```python
from build123d import *

# Parameters (mm, degrees)
SKETCH1_W           = 8.784371833
SKETCH1_H           = 3.000075643
BOSS_EXTRUDE1_DEPTH = 3.175


with BuildPart() as part:
    # Sketch1 → Boss-Extrude1 (new body)
    with BuildSketch(Plane(origin=(0, 0, 0), x_dir=(1, 0, 0), z_dir=(0, 1, 0))):
        with BuildLine():
            add(Edge.make_bspline(
                [(-28.61031783, -15.731991288), (-28.599265415, -13.470035002), (-28.589694066, -11.351623557)],
                knots=[4, 4, 4, 4.067001907, 4.067001907, 4.067001907], degree=2))
            Line((-28.61031783, -15.731991288), (-26.367380226, -15.731991288))
            Line((-26.367380226, -15.731991288), (-26.367380226, -12.731847281))
            Line((-26.367380226, -12.731847281), (-24.870018528, -12.731847281))
            Line((-24.870018528, -12.731847281), (-24.870018528, -15.731991288))
            Line((-24.870018528, -15.731991288), (-22.620949028, -15.731991288))
            Line((-22.620949028, -15.731991288), (-22.620949028, -12.731847281))
            Line((-22.620949028, -12.731847281), (-20.62449601, -12.731847281))
            Line((-20.62449601, -12.731847281), (-20.62449601, -8.731700034))
            Line((-20.62449601, -8.731700034), (-21.872234059, -8.731700034))
            Line((-21.872234059, -8.731700034), (-21.872234059, -8.631722416))
            Line((-21.872234059, -8.631722416), (-21.872234059, -6.131583692))
            Line((-21.872234059, -6.131583692), (-20.62449601, -6.131583692))
            Line((-20.62449601, -6.131583692), (-20.62449601, -2.631434402))
            Line((-20.62449601, -2.631434402), (-17.629967586, -2.631434402))
            Line((-17.629967586, -2.631434402), (-17.629967586, -6.131583692))
            Line((-17.629967586, -6.131583692), (-16.382151548, -6.131583692))
            Line((-16.382151548, -6.131583692), (-16.382151548, -8.631722416))
            Line((-16.382151548, -8.631722416), (-16.382151548, -8.731700034))
            Line((-16.382151548, -8.731700034), (-17.629967586, -8.731700034))
            Line((-17.629967586, -8.731700034), (-17.629967586, -12.731847281))
            Line((-17.629967586, -12.731847281), (-13.936374012, -12.731847281))
            Line((-13.936374012, -12.731847281), (-13.936374012, -15.731991288))
            Line((-13.936374012, -15.731991288), (-9.644077522, -15.731991288))
            Line((-9.644077522, -15.731991288), (-9.644077522, 32.969811886))
            Line((-9.644077522, 32.969811886), (-12.638791169, 32.969811886))
            Line((-12.638791169, 32.969811886), (-12.638791169, 35.969951009))
            Line((-12.638791169, 35.969951009), (-15.633504817, 35.969951009))
            Line((-15.633504817, 35.969951009), (-15.633504817, 32.969811886))
            Line((-15.633504817, 32.969811886), (-17.629967584, 32.969811886))
            Line((-17.629967584, 32.969811886), (-17.629967584, 29.869690261))
            Line((-17.629967584, 29.869690261), (-16.382151546, 29.869690261))
            Line((-16.382151546, 29.869690261), (-16.382151546, 27.369615017))
            Line((-16.382151546, 27.369615017), (-17.629967584, 27.369615017))
            Line((-17.629967584, 27.369615017), (-17.629967584, 23.569352199))
            Line((-17.629967584, 23.569352199), (-20.624496008, 23.569352199))
            Line((-20.624496008, 23.569352199), (-20.624496008, 27.369615017))
            Line((-20.624496008, 27.369615017), (-21.872234057, 27.369615017))
            Line((-21.872234057, 27.369615017), (-21.872234057, 29.869690261))
            Line((-21.872234057, 29.869690261), (-20.624496008, 29.869690261))
            Line((-20.624496008, 29.869690261), (-20.624496008, 32.969811886))
            Line((-20.624496008, 32.969811886), (-22.620949026, 32.969811886))
            Line((-22.620949026, 32.969811886), (-22.620949026, 35.969951009))
            Line((-22.620949026, 35.969951009), (-24.870018526, 35.969951009))
            Line((-24.870018526, 35.969951009), (-24.870018526, 32.969811886))
            Line((-24.870018526, 32.969811886), (-26.367380224, 32.969811886))
            Line((-26.367380224, 32.969811886), (-26.367380224, 35.969951009))
            Line((-26.367380224, 35.969951009), (-28.610317827, 35.969951009))
            Line((-28.610317827, 35.969951009), (-28.610317827, 31.489897526))
            add(Edge.make_bspline(
                [(-24.079715861, 26.005231108), (-24.142399609, 31.393191619), (-26.553744953, 31.462825341), (-28.610317827, 31.489897526)],
                knots=[6, 6, 6, 6, 7, 7, 7, 7], degree=3))
            add(Edge.make_bspline(
                [(-28.610317828, 19.811970764), (-26.367380222, 19.876359983), (-24.017041861, 20.617148519), (-24.079715861, 26.005231108)],
                knots=[5, 5, 5, 5, 6, 6, 6, 6], degree=3))
            add(Edge.make_bspline(
                [(-28.542036738, 1.284383122), (-28.493620066, 18.549619675), (-28.610317828, 19.811970764)],
                knots=[4.292555269, 4.292555269, 4.292555269, 5, 5, 5], degree=2))
            add(Edge.make_bspline(
                [(-28.542036738, 1.284383122), (-26.304598455, 1.216834034), (-24.092636702, 0.462074592), (-24.122268671, -5.143929938)],
                knots=[1.002428408, 1.002428408, 1.002428408, 1.002428408, 2, 2, 2, 2], degree=3))
            add(Edge.make_bspline(
                [(-24.122268671, -5.143929938), (-24.151883253, -10.744553605), (-26.537723417, -11.321030016), (-28.589694066, -11.351623557)],
                knots=[2, 2, 2, 2, 2.996659117, 2.996659117, 2.996659117, 2.996659117], degree=3))
        make_face()
        with Locations((-19.726124806, 7.868969519)):
            Rectangle(SKETCH1_W, SKETCH1_H, mode=Mode.SUBTRACT)
    extrude(amount=BOSS_EXTRUDE1_DEPTH)


solid = part.part
```
CAD build for the part. Positions are in the model's coordinates, mm. A direction names the side the tool comes from. Round coordinates to 2 decimals unless told otherwise and drop trailing zeros. Order: outer loops, then holes, each group sorted by start corner. A loop starts at its lowest first (then second) coordinate and runs counter-clockwise, first axis right, second up. Notation, with made-up numbers: (0.5, 86.25) - (8.5, 86.25) arc R21 cw to (8.5, 108.25) - close; hole circle Ø4 at (55, 54). An arc over 180 degrees is marked (long way). Answer as CSV lines item,"result". Start each with the question number.
1. Saw through at D-D, the plane x = -27. Count the separate pieces of the cut face and the enclosed holes in it, and give its area (3 significant figures).
2. Saw through at C-C, the plane x = -11.25. Write the cut outline in (y, z) (3 decimals).
3. Saw through at B-B, the plane x = -23.25. Write the cut outline in (y, z) (3 decimals), and give its area (3 significant figures).
4. Pull direction X, two halves, no side cores. Call faces 5 (the face through (-12, 2, 15.732)), 6 (the face through (-24.87, 2, -34)): +X half, -X half, draft (parallel to the pull), parting line (faces both ways), or undercut.
5. Saw through at A-A, the plane x = -19. Write the cut outline in (y, z) (3 decimals).
6. Tool access for faces 1 (the face through (-11, 2, -32.97)), 2 (the face through (-19, 2, -23.569)), 3 (the face through (-24.87, 2, 14)), 4 (the face through (-24.118, 2, -8)): list every direction of +Z, -Z, +X, -X, +Y, -Y with a clear straight run to the whole face (end or side of a thin tool).
7. Drill centre lines: L1, parallel to Z at x = -17.5, y = 0.6; L2, parallel to X at y = 1.45, z = 5.5; L3, parallel to Z at x = -27.5, y = 1.4. Where is each one in solid material? Low to high. Write a range as [from, to].
8. Pin check, flat tips, straight feed: pin 1 (1.5 mm diameter, centred on y = 1.5, z = -34.5, fed in from +X); pin 2 (1 mm diameter, centred on x = -17, y = 1, fed in from -Z); pin 3 (0.6 mm diameter, centred on x = -17, y = 2, fed in from +Z). Stop position of each tip, or through.
Model answer:
1,separate pieces,"3"
1,enclosed holes,"0"
1,area,"89.4 mm²"
2,outline,"(0, -32.97) - (3.175, -32.97) - (3.175, 15.732) - (0, 15.732) - close"
3,outline,"(0, -35.97) - (3.175, -35.97) - (3.175, -9.369) - (0, -9.369) - close; (0, -6.369) - (3.175, -6.369) - (3.175, 15.732) - (0, 15.732) - close"
3,area,"155 mm²"
4,face 5,"draft"
4,face 6,"undercut"
5,outline,"(0, -23.569) - (3.175, -23.569) - (3.175, -9.369) - (0, -9.369) - close; (0, -6.369) - (3.175, -6.369) - (3.175, 2.631) - (0, 2.631) - close"
6,face 1,"-Z, +X, +Y, -Y"
6,face 2,"-Z, +Y, -Y"
6,face 3,"+Z, +Y, -Y"
6,face 4,"+Y, -Y"
7,L1,"z = [-32.97, -29.87], [-27.37, -9.37], [-6.37, 6.13], [8.73, 12.73]"
7,L2,"x = [-24.13, -20.62], [-17.63, -9.64]"
7,L3,"z = [-35.97, -31.44], [-19.92, -1.19], [11.26, 15.73]"
8,pin 1,"stops at x = -12.64"
8,pin 2,"stops at z = -32.97"
8,pin 3,"stops at z = 12.73"
